Source: CAD feature listing. Evaluate the final solid. Frame: model axes, mm. Round coordinates to 2 decimals unless told otherwise and drop trailing zeros. Order: outer loops, then holes, each group sorted by start corner. A loop starts at its lowest first (then second) coordinate and runs counter-clockwise, first axis right, second up. Notation, with made-up numbers: (45.25, 26.5) - (77.25, 26.5) arc R10 cw to (77.25, 35.5) - close; hole circle Ø1 at (3.5, 84.5). An arc over 180 degrees is marked (long way). Put each result on its own line as item: value. Start each with the question number.
1) Section C-C on y = 0. Output: boundary loops of the cut face in (x, z).
2) Section B-B on x = 25. Output: boundary loops of the cut face in (y, z).
3) Section A-A on y = 15. Output: boundary loops of the cut face in (x, z), then the cut area to 3 significant figures.
4) Contact query for flat-ended pins moving along their axis: P1, Ø4, axis at x = 25, y = 15, coming from the +Z side; P2, Ø2.5, axis at x = 25, y = -15, coming from the +Z side. Output: stop coordinate, or through.
5) Section D-D on z = 7. Output: boundary loops of the cut face in (x, y).
6) Line query: probe 1 along Y at (x, z) = (25, 7.75); probe 2 along Z at (x, y) = (0, 14); probe 3 along X at (y, z) = (17, 7). Output: solid intervals per line, ascending. Write a range as [from, to].
```python
from build123d import *

# Parameters (mm, degrees)
IZIM1_W                     = 60
IZIM1_H                     = 40
IZIM1_R                     = 1.5
IZIM1_R_2                   = 8
Y_KSEKLIK_EKSTR_ZYON1_DEPTH = 18
IZIM2_R                     = 1.95
KES_EKSTR_ZYON1_DEPTH       = 28


with BuildPart() as part:
    # Çizim1 → Yükseklik-Ekstrüzyon1 (new body)
    with BuildSketch(Plane.XY):
        Rectangle(IZIM1_W, IZIM1_H)
        with Locations((-25, 15)):
            Circle(IZIM1_R, mode=Mode.SUBTRACT)
        Circle(IZIM1_R_2, mode=Mode.SUBTRACT)
        with Locations((25, 15)):
            Circle(IZIM1_R, mode=Mode.SUBTRACT)
        with Locations((25, -15)):
            Circle(IZIM1_R, mode=Mode.SUBTRACT)
        with Locations((-25, -15)):
            Circle(IZIM1_R, mode=Mode.SUBTRACT)
    extrude(amount=Y_KSEKLIK_EKSTR_ZYON1_DEPTH)

    # Çizim2 → Kes-Ekstrüzyon1 (cut)
    with BuildSketch(Plane(origin=(0, 20, 0), x_dir=(1, 0, 0), z_dir=(0, 1, 0))):
        with Locations(Location((0, -7, 0), (0, 0, 270))):
            Circle(IZIM2_R)
    extrude(amount=-KES_EKSTR_ZYON1_DEPTH, mode=Mode.SUBTRACT)


solid = part.part
```
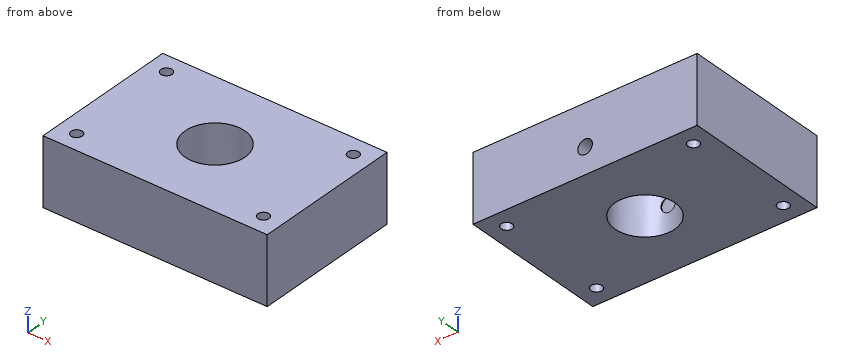
Answer sheet:
1. outline: (-30, 0) - (-8, 0) - (-8, 18) - (-30, 18) - close; (8, 0) - (30, 0) - (30, 18) - (8, 18) - close
2. outline: (-20, 0) - (-16.5, 0) - (-16.5, 18) - (-20, 18) - close; (-13.5, 0) - (13.5, 0) - (13.5, 18) - (-13.5, 18) - close; (16.5, 0) - (20, 0) - (20, 18) - (16.5, 18) - close
3. outline: (-30, 0) - (-26.5, 0) - (-26.5, 18) - (-30, 18) - close; (-23.5, 0) - (23.5, 0) - (23.5, 18) - (-23.5, 18) - close; (26.5, 0) - (30, 0) - (30, 18) - (26.5, 18) - close; hole circle Ø3.9 at (0, 7)
3. area: 960 mm^2
4. P1: z = 18
4. P2: through
5. outline: (-30, -20) - (30, -20) - (30, 20) - (1.95, 20) - (1.95, 7.76) arc R8 cw to (1.95, -7.76) - (1.95, -8) - (-1.95, -8) - (-1.95, -7.76) arc R8 cw to (-1.95, 7.76) - (-1.95, 20) - (-30, 20) - close; hole circle Ø3 at (-25, -15); hole circle Ø3 at (-25, 15); hole circle Ø3 at (25, -15); hole circle Ø3 at (25, 15)
6. probe 1: [-20, -16.5], [-13.5, 13.5], [16.5, 20]
6. probe 2: [0, 5.05], [8.95, 18]
6. probe 3: [-30, -1.95], [1.95, 30]
